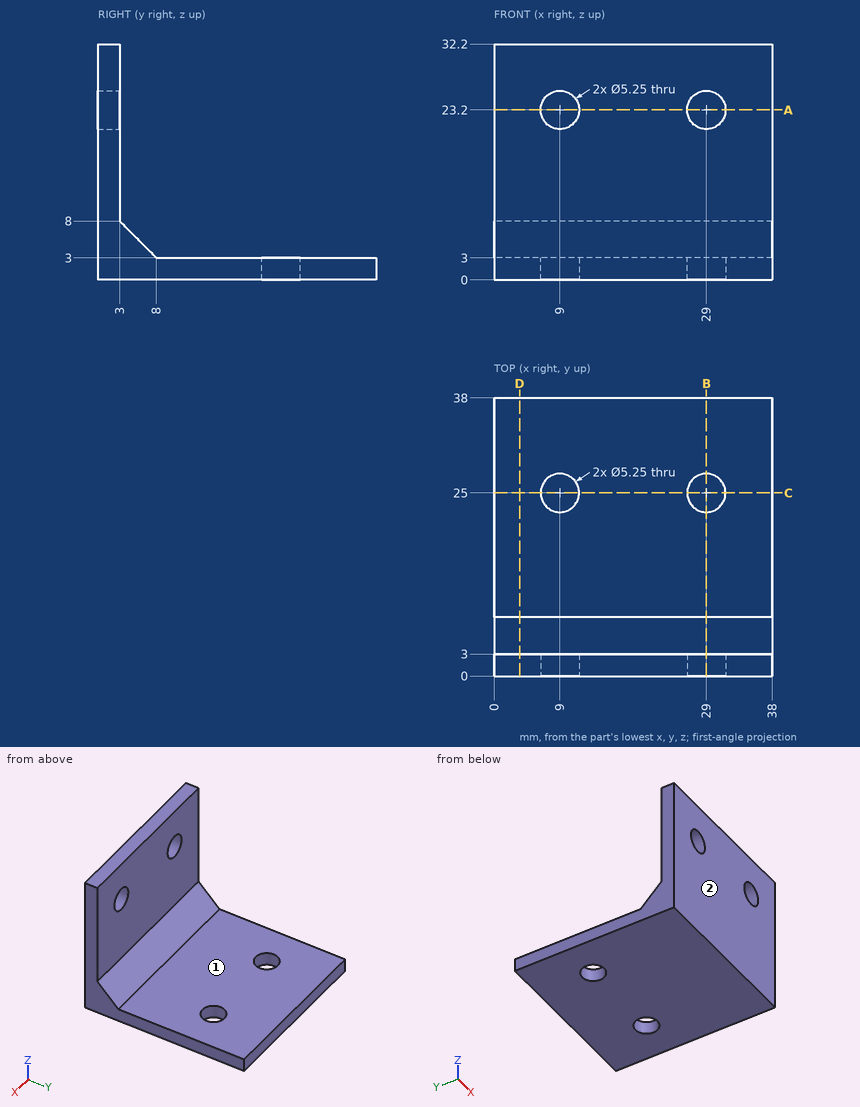
Job drawing, mm, ordinate dimensions from the low corner. One solid piece. A direction names the side the tool comes from. Give positions to 0.01 mm unless a question says otherwise; leave off trailing zeros. Loops run counter-clockwise (first coordinate to the right, second up) from the corner with the lowest first, then second, coordinate; pieces in that order, holes last. Notation, with made-up numbers: (49.5, 89.25) - (56.5, 89.25) arc R24 cw to (56.5, 119.25) - close; hole circle Ø4 at (23, 17). An arc over 180 degrees is marked (long way). Use one line per item in the form item = value.
(1) Drill centre lines: L1, parallel to X at y = 1, z = 23; L2, parallel to Z at x = 29, y = 1.05 (3 decimals); L3, parallel to Y at x = 9, z = 1.85 (3 decimals). Where is each one in solid material? Low to high.
Determined:
L1 = 0 to 6.38, 11.62 to 26.38, 31.62 to 38
L2 = 0 to 20.575, 25.825 to 32.2
L3 = 0 to 22.375, 27.625 to 38
(2) Cut at D-D (x = 3.5). Give the cut face in (y, z).
Determined:
outline = (0, 0) - (38, 0) - (38, 3) - (8, 3) - (3, 8) - (3, 32.2) - (0, 32.2) - close
(3) Cut at B-B (x = 29). Give the cut face in (y, z) (3 decimals), then the cut area to 3 significant figures.
Determined:
outline = (0, 0) - (22.375, 0) - (22.375, 3) - (8, 3) - (3, 8) - (3, 20.575) - (0, 20.575) - close; (0, 25.825) - (3, 25.825) - (3, 32.2) - (0, 32.2) - close; (27.625, 0) - (38, 0) - (38, 3) - (27.625, 3) - close
area = 183 mm^2
(4) Cut at A-A (z = 23.2). Give the cut face in (x, y) (3 decimals), then the cut area to 3 significant figures.
Determined:
outline = (0, 0) - (6.375, 0) - (6.375, 3) - (0, 3) - close; (11.625, 0) - (26.375, 0) - (26.375, 3) - (11.625, 3) - close; (31.625, 0) - (38, 0) - (38, 3) - (31.625, 3) - close
area = 82.5 mm^2
(5) Drop flat-ended pins along their axis: P1, Ø4.5, axis at x = 9, z = 23.2, coming from the +Y side; P2, Ø9, axis at x = 25.5, y = 26, coming from the +Z side; P3, Ø6, axis at x = 17, z = 7.5, coming from the -Y side; P4, Ø12, axis at x = 34, z = 13, coming from the +Y side. Give the stop position or say it passes through.
Determined:
P1 = through
P2 = 3
P3 = 0
P4 = 4
(6) 3-axis set-ups, long thin cutter, end or side, ignore diameter. For the marked faces 1 and 2: which of +Z, -Z, +X, -X, +Y, -Y reach the whole face in a straight line?
Determined:
face_1 = +Z, +X, -X, +Y
face_2 = +Z, -Z, +X, -X, -Y
